Solid Edge part; units mm, degrees
sketch "Sketch1" plane through (0, 0, 0) normal (1, 0, 0) x (0, 1, 0)
  line L0 (-22.5, -22.5) -> (22.5, -22.5)
  line L1 (22.5, -22.5) -> (22.5, 22.5)
  line L2 (22.5, 22.5) -> (-22.5, 22.5)
  line L3 (-22.5, 22.5) -> (-22.5, -22.5)
extrude "Protrusion1" add sketch "Sketch1" along normal mid plane 70
sketch "Sketch2" plane through (35, 0, 0) normal (1, 0, 0) x (0, 1, 0)
  circle A0 centre (0, 0) radius 20
extrude "Cutout1" cut sketch "Sketch2" against normal up to next
sketch "Sketch3" plane through (31, 0, 0) normal (1, 0, 0) x (0, 1, 0)
  line L0 (-20.5, -20.5) -> (20.5, -20.5)
  line L1 (20.5, -20.5) -> (20.5, 20.5)
  line L2 (20.5, 20.5) -> (-20.5, 20.5)
  line L3 (-20.5, 20.5) -> (-20.5, -20.5)
extrude "ExtrudedCutout_4" cut sketch "Sketch3" against normal blind 62
sketch "Sketch4" plane through (0, 0, 22.5) normal (0, 0, 1) x (0, -1, 0)
  line L0 (-15, -17.5) -> (15, -17.5)
  line L1 (15, -17.5) -> (15, 17.5)
  line L2 (15, 17.5) -> (-15, 17.5)
  line L3 (-15, 17.5) -> (-15, -17.5)
extrude "Cutout2" cut sketch "Sketch4" against normal up to next
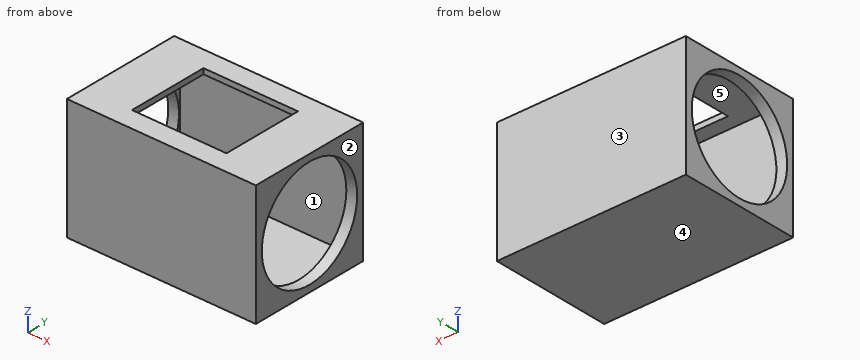
Source: CAD feature listing. Evaluate the final solid. Frame: model axes, mm. Face numbers are marked on the shaded views. A direction names the side the tool comes from. Round coordinates to 2 decimals unless told otherwise and drop trailing zeros. Loops run counter-clockwise (first coordinate to the right, second up) from the corner with the lowest first, then second, coordinate; pieces in that order, holes last. Notation, with made-up numbers: (0.25, 33.5) -> (59.25, 33.5) arc R23 ccw to (59.25, 51.5) -> close; hole circle Ø3 at (64, -40). An arc over 180 degrees is marked (long way). Answer as a JSON object with one key per item and string values. Group by question number.
Q1. Section query B-B (x = -19). Output: boundary loops of the cut face in (y, z), plus the area to 3 significant figures.
Q2. Section query D-D (y = -16). Output: boundary loops of the cut face in (x, z).
Q3. Section query C-C (z = 0). Output: boundary loops of the cut face in (x, y).
Q4. Ray query, line 1 (Z direction, x = -34.15, y = 0); line 2 (Y direction, x = -18.5, z = -9); line 3 (X direction, y = 13.5, z = 19.5). Return the intervals inside material, ascending. Write a range as from..to.
Q5. Contact query for flat-ended pins moving along their axis: P1, Ø10, axis at y = -13.5, z = -12, coming from the -X side; P2, Ø6, axis at x = 6, y = 5.5, coming from the +Z side; P3, Ø20.5, axis at y = 1, z = -4, coming from the +X side. Output: stop coordinate, or through.
Q6. Section query A-A (y = 0). Output: boundary loops of the cut face in (x, z), plus the area to 3 significant figures.
Q7. Access query for the marked faces 1 and 2. Directions: +Z, -Z, +X, -X, +Y, -Y. A direction counts if a zero-diameter tool reaches every point of the face in a straight line with its end or side. Return the directions, or none.
Q8. Mould query, pull axis Z, two halves, no side actions, for the marked faces 3, 4 and 5. Classes: pulls with the +Z half, pulls with the -Z half, needs draft (parallel to the pull), parting line crosses it, or undercut.
Completed:
{
 "1": {"outline": "(-22.5, -22.5) -> (22.5, -22.5) -> (22.5, 22.5) -> (-22.5, 22.5) -> close; hole (-20.5, -20.5) -> (20.5, -20.5) -> (20.5, 20.5) -> (-20.5, 20.5) -> close", "area": "344 mm²"},
 "2": {"outline": "(-35, -22.5) -> (35, -22.5) -> (35, -12) -> (31, -12) -> (31, -20.5) -> (-31, -20.5) -> (-31, -12) -> (-35, -12) -> close; (-35, 12) -> (-31, 12) -> (-31, 20.5) -> (31, 20.5) -> (31, 12) -> (35, 12) -> (35, 22.5) -> (-35, 22.5) -> close"},
 "3": {"outline": "(-35, -22.5) -> (35, -22.5) -> (35, -20) -> (31, -20) -> (31, -20.5) -> (-31, -20.5) -> (-31, -20) -> (-35, -20) -> close; (-35, 20) -> (-31, 20) -> (-31, 20.5) -> (31, 20.5) -> (31, 20) -> (35, 20) -> (35, 22.5) -> (-35, 22.5) -> close"},
 "4": {"line 1": "-22.5..-20, 20..22.5", "line 2": "-22.5..-20.5, 20.5..22.5", "line 3": "-35..-31, 31..35"},
 "5": {"P1": "x = -35", "P2": "z = -20.5", "P3": "through"},
 "6": {"outline": "(-35, -22.5) -> (35, -22.5) -> (35, -20) -> (31, -20) -> (31, -20.5) -> (-31, -20.5) -> (-31, -20) -> (-35, -20) -> close; (-35, 20) -> (-31, 20) -> (-31, 20.5) -> (-17.5, 20.5) -> (-17.5, 22.5) -> (-35, 22.5) -> close; (17.5, 20.5) -> (31, 20.5) -> (31, 20) -> (35, 20) -> (35, 22.5) -> (17.5, 22.5) -> close", "area": "218 mm²"},
 "7": {"face 1": "none", "face 2": "+Z, -Z, +X, +Y, -Y"},
 "8": {"face 3": "needs draft", "face 4": "pulls with the -Z half", "face 5": "undercut"}
}
